Work out the finished part from the listing and answer in its coordinate system (mm). Give positions to 0.01 mm unless a question says otherwise; leave off trailing zeros. Write each loop counter-clockwise with the first axis right and the second up, starting at its lowest first coordinate (ties: lowest second). Pieces come first, ordered by that corner, then holes.
1) Given pin 1 Ø5 at (x, y) = (6, -3.5) entering from -Z, flat-ended and moving along its own axis, determine where the tip first touches the part or whether it passes through.
2) Find section C-C (y = -5.75). Determine the outline of the cut face in (x, z).
3) Find section A-A (y = -19.25). Determine the outline of the cut face in (x, z).
4) Straight lines are drawn through the part: probe 1 along Y at (x, z) = (5.75, 1.05); probe 2 along Y at (x, z) = (19.25, 0.6); probe 3 along Y at (x, z) = (2.75, 0.7). For each, find the intervals that lie inside material, in ascending order.
5) Find section B-B (z = 0.55). Determine the outline of the cut face in (x, y).
```python
from build123d import *

# Parameters (mm, degrees)
SKETCH1_W                      = 25.4
SKETCH1_H                      = 25.4
BOSS_EXTRUDE1_DEPTH            = 1.27
MOUNTING_HOLES_FOR_MOTOR_REACH = 37.943
SKETCH8_R                      = 1.8415
FILLET2_R                      = 8.89


with BuildPart() as part:
    # Sketch1 → Boss-Extrude1 (new body)
    with BuildSketch(Plane.XY):
        with Locations((12.7, -12.7)):
            Rectangle(SKETCH1_W, SKETCH1_H)
    extrude(amount=BOSS_EXTRUDE1_DEPTH)

    # Sketch8 → Mounting Holes for Motor (cut, up to next)
    with BuildSketch(Plane.XY.offset(1.27), mode=Mode.PRIVATE) as mounting_holes_for_motor_sk1:
        with Locations((20.557724106, -4.842275894)):
            Circle(SKETCH8_R)
    mounting_holes_for_motor_tool1 = extrude(mounting_holes_for_motor_sk1.sketch, amount=-MOUNTING_HOLES_FOR_MOTOR_REACH, mode=Mode.PRIVATE) & part.part
    # Sketch8 → Mounting Holes for Motor (cut, up to next)
    with BuildSketch(Plane.XY.offset(1.27), mode=Mode.PRIVATE) as mounting_holes_for_motor_sk2:
        with Locations((4.842275894, -4.842275894)):
            Circle(SKETCH8_R)
    mounting_holes_for_motor_tool2 = extrude(mounting_holes_for_motor_sk2.sketch, amount=-MOUNTING_HOLES_FOR_MOTOR_REACH, mode=Mode.PRIVATE) & part.part
    # Sketch8 → Mounting Holes for Motor (cut, up to next)
    with BuildSketch(Plane.XY.offset(1.27), mode=Mode.PRIVATE) as mounting_holes_for_motor_sk3:
        with Locations((4.842275894, -20.557724106)):
            Circle(SKETCH8_R)
    mounting_holes_for_motor_tool3 = extrude(mounting_holes_for_motor_sk3.sketch, amount=-MOUNTING_HOLES_FOR_MOTOR_REACH, mode=Mode.PRIVATE) & part.part
    # Sketch8 → Mounting Holes for Motor (cut, up to next)
    with BuildSketch(Plane.XY.offset(1.27), mode=Mode.PRIVATE) as mounting_holes_for_motor_sk4:
        with Locations((20.557724106, -20.557724106)):
            Circle(SKETCH8_R)
    mounting_holes_for_motor_tool4 = extrude(mounting_holes_for_motor_sk4.sketch, amount=-MOUNTING_HOLES_FOR_MOTOR_REACH, mode=Mode.PRIVATE) & part.part
    add(mounting_holes_for_motor_tool1.solids().sort_by_distance((20.557724, -4.842276, 1.27))[0], mode=Mode.SUBTRACT)
    add(mounting_holes_for_motor_tool2.solids().sort_by_distance((4.842276, -4.842276, 1.27))[0], mode=Mode.SUBTRACT)
    add(mounting_holes_for_motor_tool3.solids().sort_by_distance((4.842276, -20.557724, 1.27))[0], mode=Mode.SUBTRACT)
    add(mounting_holes_for_motor_tool4.solids().sort_by_distance((20.557724, -20.557724, 1.27))[0], mode=Mode.SUBTRACT)

    # Fillet2
    fillet2_edges = [part.edges().sort_by_distance(p)[0] for p in [
        (0, 0, 0.635),
        (25.4, 0, 0.635),
        (25.4, -25.4, 0.635),
        (0, -25.4, 0.635),
    ]]
    fillet(fillet2_edges, radius=FILLET2_R)


solid = part.part
```
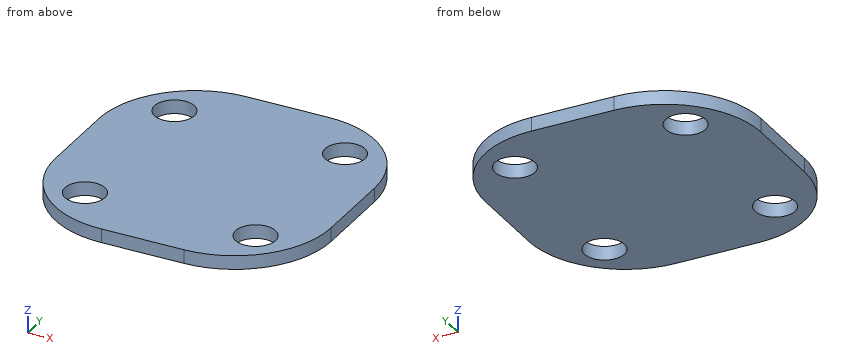
Results:
1. pin 1: stops at z = 0
2. outline: (0.57, 0) - (3.24, 0) - (3.24, 1.27) - (0.57, 1.27) - close; (6.44, 0) - (18.96, 0) - (18.96, 1.27) - (6.44, 1.27) - close; (22.16, 0) - (24.83, 0) - (24.83, 1.27) - (22.16, 1.27) - close
3. outline: (0.43, 0) - (3.55, 0) - (3.55, 1.27) - (0.43, 1.27) - close; (6.14, 0) - (19.26, 0) - (19.26, 1.27) - (6.14, 1.27) - close; (21.85, 0) - (24.97, 0) - (24.97, 1.27) - (21.85, 1.27) - close
4. probe 1: y = -24.83 to -22.16, -18.96 to -6.44, -3.24 to -0.57
4. probe 2: y = -24.97 to -21.85, -19.26 to -6.14, -3.55 to -0.43
4. probe 3: y = -22.94 to -2.46
5. outline: (0, -16.51) arc R8.89 ccw to (8.89, -25.4) - (16.51, -25.4) arc R8.89 ccw to (25.4, -16.51) - (25.4, -8.89) arc R8.89 ccw to (16.51, 0) - (8.89, 0) arc R8.89 ccw to (0, -8.89) - close; hole circle Ø3.68 at (4.84, -20.56); hole circle Ø3.68 at (4.84, -4.84); hole circle Ø3.68 at (20.56, -20.56); hole circle Ø3.68 at (20.56, -4.84)
